```python
from build123d import *

# Parameters (mm, degrees)
EXTRUDE002_DEPTH = 20
SKETCH003_R      = 10
EXTRUDE_DEPTH    = 10
SKETCH_W         = 45
SKETCH_H         = 45
PAD_DEPTH        = 5


with BuildPart() as extrude002:
    # Sketch008 (on Face1 of CopyExtrude) → Extrude002 (new body)
    with BuildSketch(Plane(origin=(0, 0, -10), x_dir=(1, 0, 0), z_dir=(0, 0, -1))):
        with BuildLine():
            ThreePointArc((20.5, 19.035898), (26.5, 22.5), (20.5, 25.964102))
            Line((20.5, 25.964102), (20.5, 19.035898))
        make_face()
    extrude(amount=-EXTRUDE002_DEPTH)


with BuildPart() as valec:
    # Sketch003 → Extrude (new body)
    with BuildSketch(Plane(origin=(0, 0, 0), x_dir=(1, 0, 0), z_dir=(0, 0, -1))):
        with Locations((22.5, 22.5)):
            Circle(SKETCH003_R)
    extrude(amount=EXTRUDE_DEPTH)


with BuildPart() as obj1:
    # Sketch → Pad (new body)
    with BuildSketch(Plane.XY):
        with Locations((22.5, -22.5)):
            Rectangle(SKETCH_W, SKETCH_H)
    extrude(amount=PAD_DEPTH)

    # Fusion: union Valec
    add(valec.part)

    # Cut: cut Extrude002
    add(extrude002.part, mode=Mode.SUBTRACT)


solid = obj1.part
```
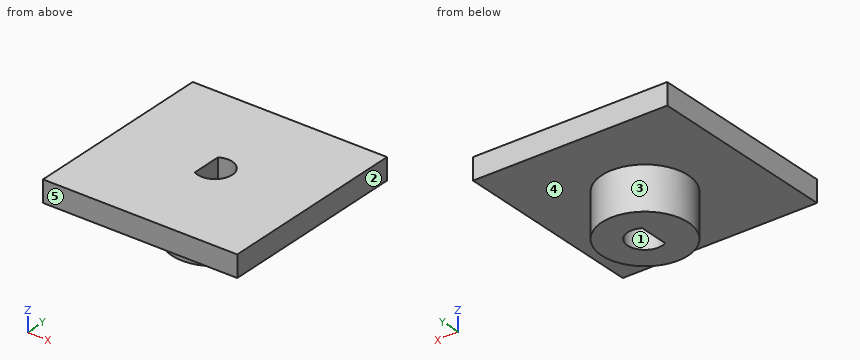
Source: CAD feature listing. Evaluate the final solid. Frame: model axes, mm. Face numbers are marked on the shaded views. A direction names the side the tool comes from. Coordinates: 2 decimals unless noted, no trailing zeros. Loops run counter-clockwise (first coordinate to the right, second up) from the corner with the lowest first, then second, coordinate; pieces in that order, holes last. Notation, with made-up numbers: M 5,28 L 21,28 A28 ccw 21,65 Z; hole C -32,74 d11. An arc over 180 degrees is marked long. Use a Markdown table: item, result. Add a question column.
Q1. Section query A-A, the plane x = 22.5. Return loops of the section in (y, z).
Q2. Section query D-D, the plane z = -6. Return loops of the section in (x, y).
Q3. Material intervals for L1, parallel to X at y = -22.5, z = -7; L2, parallel to Y at x = 22.5, z = -5.5; L3, parallel to Y at x = 22.5, z = 1, sorted ascending.
Q4. First-contact query: pin 1 (8 mm diameter, centred on y = -6, z = -5, fed in from +X); pin 2 (8 mm diameter, centred on x = 26, z = -6, fed in from -Y); pin 3 (6 mm diameter, centred on x = 23.5, y = -35.5, fed in from -Z). Flat tips, straight axial feed; report the tip coordinate or a pass-through.
Q5. Access query for the marked faces 4 and 5. Directions: +Z, -Z, +X, -X, +Y, -Y. A direction counts if a zero-diameter tool reaches every point of the face in a straight line with its end or side. Return the directions, or none.
Q6. Section query C-C, the plane y = -14.5. Return loops of the section in (x, z).
Q7. Draft query along Y for the marked faces 1, 2 and 3. Return one class per face: pulls with the +Y half, pulls with the -Y half, needs draft (parallel to the pull), parting line crosses it, or undercut.
Q8. Section query B-B, the plane y = -22.5. Return loops of the section in (x, z).
Result:
| question | item | result |
|---|---|---|
| 1 | outline | M -45,0 L -32.5,0 L -32.5,-10 L -26.5,-10 L -26.5,5 L -45,5 Z; M -18.5,-10 L -12.5,-10 L -12.5,0 L 0,0 L 0,5 L -18.5,5 Z |
| 2 | outline | C 22.5,-22.5 d20; hole M 20.5,-25.96 A4 ccw long 20.5,-19.04 Z |
| 3 | L1 | x = 12.5 to 20.5, 26.5 to 32.5 |
| 3 | L2 | y = -32.5 to -26.5, -18.5 to -12.5 |
| 3 | L3 | y = -45 to -26.5, -18.5 to 0 |
| 4 | pin 1 | passes through |
| 4 | pin 2 | stops at y = -32.5 |
| 4 | pin 3 | stops at z = 0 |
| 5 | face 4 | -Z |
| 5 | face 5 | +Z, -Z, +X, -X, -Y |
| 6 | outline | M 0,0 L 16.5,0 L 16.5,-10 L 28.5,-10 L 28.5,0 L 45,0 L 45,5 L 0,5 Z |
| 7 | face 1 | undercut |
| 7 | face 2 | needs draft |
| 7 | face 3 | parting line crosses it |
| 8 | outline | M 0,0 L 12.5,0 L 12.5,-10 L 20.5,-10 L 20.5,5 L 0,5 Z; M 26.5,-10 L 32.5,-10 L 32.5,0 L 45,0 L 45,5 L 26.5,5 Z |
